Model file for the job. Use its own axes, mm. Face numbers are marked on the shaded views. Coordinates: 2 decimals unless noted, no trailing zeros. Order: outer loops, then holes, each group sorted by start corner. A loop starts at its lowest first (then second) coordinate and runs counter-clockwise, first axis right, second up. Notation, with made-up numbers: (49.5, 13.25) - (55.5, 13.25) arc R24 cw to (55.5, 52.25) - close; hole circle Ø7 at (32, 79). An arc over 180 degrees is marked (long way). Put each result on its own line as item: value. Start each with the question number.
```python
from build123d import *

# Parameters (mm, degrees)
PVC_R               = 57
PVC_R_2             = 51
BOSS_EXTRUDE1_DEPTH = 76.2
CUT_EXTRUDE1_START  = -110
CUT_EXTRUDE1_DEPTH  = 100


with BuildPart() as part:
    # PVC → Boss-Extrude1 (new, symmetric)
    with BuildSketch(Plane(origin=(0, 0, 0), x_dir=(1, 0, 0), z_dir=(0, 1, 0))):
        with Locations(Location((0, 0, 0), (0, 0, 90))):
            Circle(PVC_R)
        with Locations(Location((0, 0, 0), (0, 0, 90))):
            Circle(PVC_R_2, mode=Mode.SUBTRACT)
    extrude(amount=BOSS_EXTRUDE1_DEPTH, both=True)

    # Sketch1 → Cut-Extrude1 (cut)
    with BuildSketch(Plane.XZ.offset(76.2).offset(CUT_EXTRUDE1_START)):
        with BuildLine():
            Line((0, 0), (43.531515848, 36.796835842))
            ThreePointArc((43.531515848, 36.796835842), (57, 0), (43.531515848, -36.796835842))
            Line((43.531515848, -36.796835842), (0, 0))
        make_face()
    extrude(amount=CUT_EXTRUDE1_DEPTH, mode=Mode.SUBTRACT)


solid = part.part
```
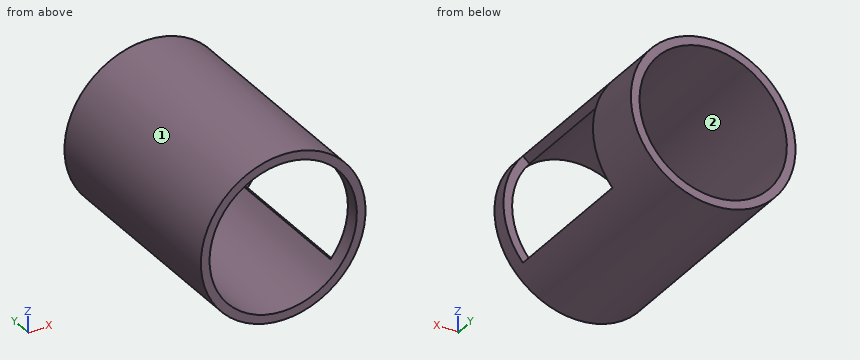
Item 1: Slice it at D-D, the plane y = 4.5. Give the cut face in (x, z), plus the area to 3 significant figures.
Item 2: Wall check: line 1 along X through (y, z) = (59, -38.5); line 2 along Z through (x, y) = (0.5, -49.5); line 3 along X through (y, z) = (-45, 0). Give the ranges that are in metal, low to high.
Item 3: Pull direction Z, two halves, no side cores. Call the marked faces 1 and 2: pulls with the +Z half, pulls with the -Z half, needs draft (parallel to the pull), parting line crosses it, or undercut.
Item 4: Slice it at C-C, the plane z = -44.5. Give the cut face in (x, y).
Item 5: Flat gauge pins, fed straight in: pin 1 Ø5 at (x, y) = (-25, -60) entering from +Z; pin 2 Ø3 at (y, z) = (-30, 1) entering from +X; pin 3 Ø14.5 at (x, z) = (49.5, 4) entering from +Y; pin 4 Ø1 at (x, y) = (36.5, -33.5) entering from +Z. Where does each tip first touch, or does it go through?
Item 6: Slice it at B-B, the plane x = 0. Give the cut face in (y, z).
Item 7: Slice it at A-A, the plane z = 0. Give the cut face in (x, y).
Here are the results:
1. outline: (38.95, -32.92) arc R51 cw (long way) to (38.95, 32.92) - (43.53, 36.8) arc R57 ccw (long way) to (43.53, -36.8) - close
1. area: 1,580 mm^2
2. line 1: x = -42.03 to -33.45, 33.45 to 42.03
2. line 2: z = -57 to -51, 51 to 57
2. line 3: x = -57 to -51
3. face 1: parting line crosses it
3. face 2: undercut
4. outline: (-35.62, -76.2) - (-24.91, -76.2) - (-24.91, 76.2) - (-35.62, 76.2) - close; (24.91, -76.2) - (35.62, -76.2) - (35.62, 76.2) - (24.91, 76.2) - close
5. pin 1: stops at z = 52.37
5. pin 2: stops at x = -50.94
5. pin 3: stops at y = 76.2
5. pin 4: stops at z = 44.19
6. outline: (-76.2, -57) - (76.2, -57) - (76.2, -51) - (-76.2, -51) - close; (-76.2, 51) - (76.2, 51) - (76.2, 57) - (-76.2, 57) - close
7. outline: (-57, -76.2) - (-51, -76.2) - (-51, 76.2) - (-57, 76.2) - close; (51, -76.2) - (57, -76.2) - (57, -66.2) - (51, -66.2) - close; (51, 33.8) - (57, 33.8) - (57, 76.2) - (51, 76.2) - close
